```python
from build123d import *

# Parameters (mm, degrees)
F0_R     = 5
F1_DEPTH = 4
F2_W     = 5.6
F2_H     = 5.6
F3_DEPTH = 2
F4_R     = 5
F5_DEPTH = 4
F6_R     = 1.1936420452
F7_DEPTH = 10.001
F8_R     = 2


with BuildPart() as f1:
    # F0 (on Top) → F1 (new body)
    with BuildSketch(Plane.XY):
        Circle(F0_R)
    extrude(amount=F1_DEPTH)

    # F2 (on face) → F3 (join)
    with BuildSketch(Plane.XY.offset(4)):
        with Locations((-0.0721134877, -0.062788504)):
            Rectangle(F2_W, F2_H)
    extrude(amount=F3_DEPTH)

    # F4 (on face) → F5 (join)
    with BuildSketch(Plane.XY.offset(6)):
        Circle(F4_R)
    extrude(amount=F5_DEPTH)

    # F6 (on face) → F7 (cut, through all)
    with BuildSketch(Plane.XY.offset(10)):
        Circle(F6_R)
    extrude(amount=-F7_DEPTH, mode=Mode.SUBTRACT)

    # F8
    f8_edges = [f1.edges().sort_by_distance(p)[0] for p in [
        (-5, 0, 10),
    ]]
    fillet(f8_edges, radius=F8_R)


solid = f1.part
```
Check sheet for the modelled part. Datum: model origin and axes. Units: mm. A direction names the side the tool comes from. Give positions to 0.01 mm unless a question says otherwise; leave off trailing zeros. Write each loop counter-clockwise with the first axis right and the second up, starting at its lowest first coordinate (ties: lowest second). Pieces come first, ordered by that corner, then holes.
Item 1: Draft check along Z on faces 5 (the face through (0, 2.737, 5)), 6 (the face through (1, -1, 0)), 7 (the face through (-1.08, -4.88, 6.99)). Enter one of: released by +Z, released by -Z, zero draft, split by the parting line, or undercut.
Item 2: Cross-section at A-A (x = 0). Enter the section's corners in (y, z), and give its area (3 significant figures).
Item 3: Cross-section at D-D (z = 8.5). Enter the section's corners in (x, y), and give its area (3 significant figures).
Item 4: Cross-section at B-B (y = 0). Enter the section's corners in (x, z), and give its area (3 significant figures).
Item 5: Access from +Z, -Z, +X, -X, +Y, -Y to the whole of each face (thin tool, end or side, straight path). Record for faces 1 (the face through (2.728, 0, 5)), 2 (the face through (-2.872, 0, 5)), 3 (the face through (3, 0, 6)), 4 (the face through (0, -2.863, 5)).
Item 6: Cross-section at C-C (z = 2). Enter the section's corners in (x, y), and give its area (3 significant figures).
Item 7: Scan lines: L1, parallel to Y at x = 0, z = 7.25; L2, parallel to Y at x = 0, z = 5.75; L3, parallel to Z at x = -2, y = 3.75. Record each from-to range of solid material in increasing order.
Item 8: Gauge pin test, flat ends, axial feed: pin 1 (4 mm diameter, centred on y = -3.5, z = 8.5, fed in from -X); pin 2 (0.6 mm diameter, centred on y = -0.5, z = 5, fed in from -X); pin 3 (1.6 mm diameter, centred on x = 1, z = 5, fed in from -Y). Record the tip position at first contact, or that the pin passes through.
Report:
1. face 5: undercut
1. face 6: released by -Z
1. face 7: zero draft
2. outline: (-5, 0) - (-1.19, 0) - (-1.19, 10) - (-3, 10) arc R2 ccw to (-5, 8) - (-5, 6) - (-2.86, 6) - (-2.86, 4) - (-5, 4) - close; (1.19, 0) - (5, 0) - (5, 4) - (2.74, 4) - (2.74, 6) - (5, 6) - (5, 8) arc R2 ccw to (3, 10) - (1.19, 10) - close
2. area: 65.6 mm2
3. outline: circle Ø9.87 at (0, 0); hole circle Ø2.39 at (0, 0)
3. area: 72.1 mm2
4. outline: (-5, 0) - (-1.19, 0) - (-1.19, 10) - (-3, 10) arc R2 ccw to (-5, 8) - (-5, 6) - (-2.87, 6) - (-2.87, 4) - (-5, 4) - close; (1.19, 0) - (5, 0) - (5, 4) - (2.73, 4) - (2.73, 6) - (5, 6) - (5, 8) arc R2 ccw to (3, 10) - (1.19, 10) - close
4. area: 65.6 mm2
5. face 1: +X, +Y, -Y
5. face 2: -X, +Y, -Y
5. face 3: none
5. face 4: +X, -X, -Y
6. outline: circle Ø10 at (0, 0); hole circle Ø2.39 at (0, 0)
6. area: 74.1 mm2
7. L1: y = -5 to -1.19, 1.19 to 5
7. L2: y = -2.86 to -1.19, 1.19 to 2.74
7. L3: z = 0 to 4, 6 to 9.56
8. pin 1: stops at x = -4.75
8. pin 2: stops at x = -2.87
8. pin 3: stops at y = -2.86
